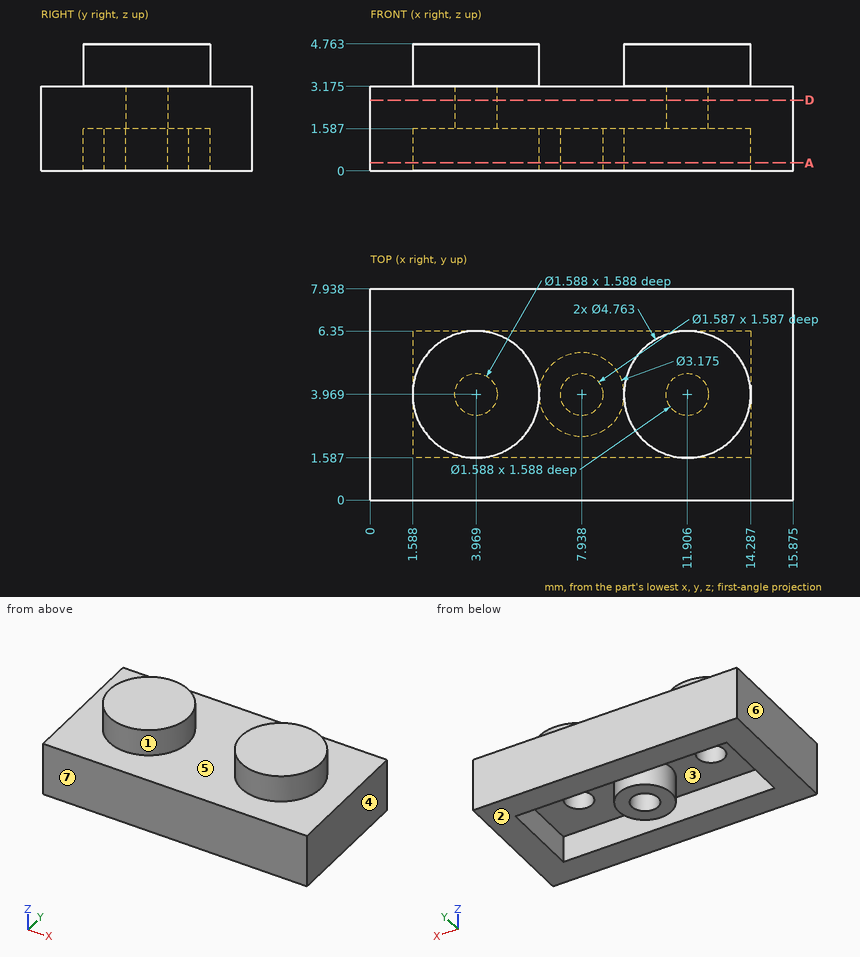
Geometry: see drawing. Coordinates: mm, zero at the bounding-box minimum. A direction names the side the tool comes from. Coordinates: 2 decimals unless noted, no trailing zeros. Loops run counter-clockwise (first coordinate to the right, second up) from the corner with the lowest first, then second, coordinate; pieces in that order, holes last. Notation, with made-up numbers: (47.25, -26.75) -> (53.25, -26.75) arc R20 cw to (53.25, -19.75) -> close; hole circle Ø6 at (35.5, 59.5). An arc over 180 degrees is marked (long way). Write item = value, one per line. Start each with the question number.
Item 1: Mould query, pull axis X, two halves, no side actions, for the marked faces 4, 5, 6 and 7. Classes: pulls with the +X half, pulls with the -X half, needs draft (parallel to the pull), parting line crosses it, or undercut.
Item 2: Cut plane A-A, the plane z = 0.3. Count the separate pieces of the cut face and the enclosed holes in it.
Item 3: First-contact query: P1, Ø1.7, axis at x = 12, y = 4.5, coming from the -Z side; P2, Ø1, axis at x = 12, y = 1, coming from the +Z side (1 decimal); P3, Ø1.3, axis at x = 3.97, y = 3.97, coming from the -Z side (1 decimal). Flat tips, straight axial feed; report the tip coordinate or a pass-through.
Item 4: Material intervals for line 1 (Y direction, x = 13.5, z = 0.5); line 2 (Z direction, x = 15.25, y = 7.75) (1 decimal); line 3 (X direction, y = 6, z = 1.5) (1 decimal), sorted ascending.
Item 5: Reachability of the marked faces 1, 2 and 3 from +Z, -Z, +X, -X, +Y, -Y: full face, straight path, thin tool, end or side. Return the list, or none.
Item 6: Cut plane D-D, the plane z = 2.65. Return loops of the section in (x, y) (1 decimal), plus the area to 3 significant figures.
Ans:
q1.face_4 = pulls with the +X half
q1.face_5 = undercut
q1.face_6 = pulls with the -X half
q1.face_7 = needs draft
q2.separate_pieces = 2
q2.enclosed_holes = 2
q3.P1 = 1.59
q3.P2 = 3.2
q3.P3 = 3.2
q4.line_1 = 0 to 1.59, 6.35 to 7.94
q4.line_2 = 0 to 3.2
q4.line_3 = 0 to 1.6, 14.3 to 15.9
q5.face_1 = +Z
q5.face_2 = -Z, +X, -X, +Y, -Y
q5.face_3 = -Z
q6.outline = (0, 0) -> (15.9, 0) -> (15.9, 7.9) -> (0, 7.9) -> close; hole circle Ø1.6 at (4, 4); hole circle Ø1.6 at (11.9, 4)
q6.area = 122 mm²
